Check sheet for the modelled part. Datum: model origin and axes. Units: mm. Face numbers are marked on the shaded views. Give positions to 0.01 mm unless a question says otherwise; leave off trailing zeros. Order: outer loops, then holes, each group sorted by start corner. A loop starts at its lowest first (then second) coordinate and runs counter-clockwise, first axis right, second up. Notation, with made-up numbers: M 70.5,16 L 103.5,16 A29 cw 103.5,50 Z; hole C 55,-19.75 d1. An arc over 180 degrees is marked long. Answer in a Markdown table with one row per item. Add a question column.
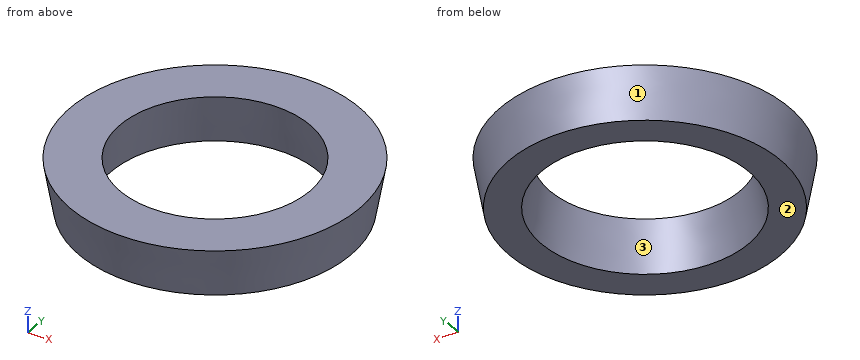
from build123d import *

# Parameters (mm, degrees)
SKETCH_1_3_R    = 29.142907565
SKETCH_1_3_R_2  = 19.142907565
EXTRUDE_1_DEPTH = 10
EXTRUDE_1_DRAFT = -10


with BuildPart() as part:
    # Эскиз1<3> → Бобышка-Вытянуть1 (with draft: the straight prism first)
    with BuildSketch(Plane.XY):
        Circle(SKETCH_1_3_R)
        Circle(SKETCH_1_3_R_2, mode=Mode.SUBTRACT)
    extrude(amount=-EXTRUDE_1_DEPTH)
    # Бобышка-Вытянуть1: the draft: its side faces are tilted about the plane it starts from
    extrude_1_sides = [part.faces().sort_by_distance(p)[0] for p in [
        (-29.142907565, 0, -5),
        (-19.142907565, 0, -5),
    ]]
    draft(extrude_1_sides, Plane.XY, EXTRUDE_1_DRAFT)


solid = part.part
Q1. Cross-section at D-D (z = -1). Record the boundary of the cut face in (x, y).
Q2. Go/stop test with flat-tipped pins: pin 1 (5 mm diameter, centred on y = -23, z = -1, fed in from +X); pin 2 (4 mm diameter, centred on y = -15.5, z = -5, fed in from -X); pin 3 (4 mm diameter, centred on x = -13, z = -2, fed in from -Y). Record where each tip stops, or that it passes through.
Q3. Cross-section at A-A (y = 0). Record the boundary of the cut face in (x, z), and give its area (3 significant figures).
Q4. Thickness scan on probe 1 along Y at (x, z) = (17, -8.5); probe 2 along Y at (x, z) = (14, -1); probe 3 along X at (y, z) = (-2, -8.75). Record the ranges inside material, lowest first.
Q5. Draft check along Y on the marked faces 1, 2 and 3. Enter one of: pulls with the +Y half, pulls with the -Y half, needs draft (parallel to the pull), parting line crosses it, or undercut.
Q6. Cross-section at C-C (z = -5.5). Record the boundary of the cut face in (x, y), and give its area (3 significant figures).
Values follow:
| question | item | result |
|---|---|---|
| 1 | outline | C 0,0 d57.93; hole C 0,0 d38.64 |
| 2 | pin 1 | x = 20.54 |
| 2 | pin 2 | x = -24.9 |
| 2 | pin 3 | y = -26.69 |
| 3 | outline | M -29.14,0 L -27.38,-10 L -20.91,-10 L -19.14,0 Z; M 19.14,0 L 20.91,-10 L 27.38,-10 L 29.14,0 Z |
| 3 | area | 165 mm² |
| 4 | probe 1 | -21.8 to -11.71, 11.71 to 21.8 |
| 4 | probe 2 | -25.36 to -13.31, 13.31 to 25.36 |
| 4 | probe 3 | -27.53 to -20.59, 20.59 to 27.53 |
| 5 | face 1 | parting line crosses it |
| 5 | face 2 | needs draft |
| 5 | face 3 | undercut |
| 6 | outline | C 0,0 d56.35; hole C 0,0 d40.23 |
| 6 | area | 1,220 mm² |
